Here's how the part is built. I have some questions about the finished solid (model axes, mm). A direction names the side the tool comes from. Round coordinates to 2 decimals unless told otherwise and drop trailing zeros. Loops run counter-clockwise (first coordinate to the right, second up) from the corner with the lowest first, then second, coordinate; pieces in that order, holes last. Notation, with made-up numbers: M -11.75,46.25 L 34.25,46.25 A23 ccw 34.25,82.25 Z; hole C 57,84 d6. An arc over 180 degrees is marked long. Use a Markdown table: item, result.
Autodesk Inventor part; units mm, degrees
ref_plane "YZ Plane" through (0, 0, 0) normal (1, 0, 0) x (0, 1, 0)
ref_plane "XZ Plane" through (0, 0, 0) normal (0, 1, 0) x (-1, 0, 0)
ref_plane "XY Plane" through (0, 0, 0) normal (0, 0, 1) x (1, 0, 0)
sketch "Sketch1" plane through (0, 0, 0) normal (0, 1, 0) x (-1, 0, 0)
  line L0 (6.6, -20) -> (-6.6, -20)
  line L1 (-6.6, -20) -> (-6.6, 20)
  line L2 (-6.6, 20) -> (6.6, 20)
  line L3 (6.6, 20) -> (6.6, -20)
  point P0 (0, 0)
  point P1 (0, -20)
  point P2 (-6.6, 0)
  dimension "d0" = 13.2
  dimension "d1" = 40
extrude "Extrusion1" add sketch "Sketch1" along normal blind 4.5
sketch "Sketch2" plane through (0, 0, 0) normal (0, -1, 0) x (1, 0, 0)
  line L0 (6.6, 20) -> (6.6, -20)
  circle A0 centre (6.6, 0) radius 2.05
  line L1 (-6.6, -20) -> (-6.6, 20)
  circle A1 centre (-6.6, 0) radius 2.05
  circle A2 centre (6.6, 0) radius 3.5
  circle A3 centre (-6.6, 0) radius 3.5
  point P0 (0, 0)
  dimension "d4" = 4.1
  dimension "d5" = 7
extrude "Extrusion2" add sketch "Sketch2" against normal blind 4.5
extrude "Extrusion3" cut sketch "Sketch2" against normal blind 3.1 contours A0 L0 | L0 A0 | A1 L1 | L1 A1
fillet "Fillet1" radius 2 8 edges at (6.6, 2.25, -20) (-6.6, 2.25, -20) (6.6, 2.25, 20) (-6.6, 2.25, 20) (6.6, 2.25, -3.5) (6.6, 2.25, 3.5) (-6.6, 2.25, -3.5) (-6.6, 2.25, 3.5)
fillet "Fillet2" radius 0.5 24 edges at (-6.6, 0, -11.5617) (-6.0142, 0, -19.4142) (0, 0, -20) (6.0142, 0, -19.4142) (6.6, 0, -11.5617) (10.1, 0, 0) (6.0142, 0, 19.4142) (6.6, 0, 11.5617) (0, 0, 20) (-6.0142, 0, 19.4142) (-6.6, 0, 11.5617) (-10.1, 0, 0) (-6.0142, 4.5, -19.4142) (-6.0142, 4.5, 19.4142) (-6.6, 4.5, 11.5617) (0, 4.5, 20) (6.0142, 4.5, 19.4142) (6.6, 4.5, 11.5617) (6.0142, 4.5, -19.4142) (10.1, 4.5, 0) (6.6, 4.5, -11.5617) (0, 4.5, -20) (-6.6, 4.5, -11.5617) (-10.1, 4.5, 0)
chamfer "Chamfer1" distance 0.25 angle 45 2 edges at (-8.65, 0, 0) (4.55, 0, 0)
properties part number "FuselageLock"
1. Imagine slicing it at A-A, the plane y = 2.55. Write out the boundary of the cut face in (x, z), then the cut area to 3 significant figures.
Answer sheet:
| item | result |
|---|---|
| outline | M -7.87,-3.26 A2 cw -6.6,-5.12 L -6.6,-18 A2 ccw -4.6,-20 L 4.6,-20 A2 ccw 6.6,-18 L 6.6,-5.12 A2 cw 7.87,-3.26 A3.5 ccw 7.87,3.26 A2 cw 6.6,5.12 L 6.6,18 A2 ccw 4.6,20 L -4.6,20 A2 ccw -6.6,18 L -6.6,5.12 A2 cw -7.87,3.26 A3.5 ccw Z; hole C -6.6,0 d4.1; hole C 6.6,0 d4.1 |
| area | 538 mm2 |
2. For pin 1 Ø1.2 at (x, z) = (6, 1) entering from -Y; pin 2 Ø1 at (y, z) = (1.5, -12.5) entering from -X; pin 3 Ø4.5 at (x, z) = (6.6, 0) entering from -Y, each with a flat end and sliding along its axis, tell me the tip position at first contact or that it passes through.
Answer sheet:
| item | result |
|---|---|
| pin 1 | y = 3.1 |
| pin 2 | x = -6.6 |
| pin 3 | y = 0.05 |
3. Which directions (+Z, -Z, +X, -X, +Y, -Y) give clear straight access to the entire face, cutting with the end or side of a thin tool? Please do faces 4 (the face through (6.6, 2, 11)), 5 (the face through (0, 4.5, 0)), 6 (the face through (4.55, 1.66, 0.09)).
Answer sheet:
| item | result |
|---|---|
| face 4 | +Z, +X, +Y, -Y |
| face 5 | +Z, -Z, +X, -X, +Y |
| face 6 | -Y |
4. Imagine slicing it at C-C, the plane z = 5.5. Write out the boundary of the cut face in (x, y), then the cut area to 3 significant figures.
Answer sheet:
| item | result |
|---|---|
| outline | M -6.6,0.5 A0.5 ccw -6.1,0 L 6.1,0 A0.5 ccw 6.6,0.5 L 6.6,4 A0.5 ccw 6.1,4.5 L -6.1,4.5 A0.5 ccw -6.6,4 Z |
| area | 59.2 mm2 |
5. Imagine slicing it at B-B, the plane z = 0. Write out the boundary of the cut face in (x, y), then the cut area to 3 significant figures.
Answer sheet:
| item | result |
|---|---|
| outline | M -10.1,0.5 A0.5 ccw -9.6,0 L -8.9,0 L -8.65,0.25 L -8.65,3.1 L -4.55,3.1 L -4.55,0.25 L -4.3,0 L 4.3,0 L 4.55,0.25 L 4.55,3.1 L 8.65,3.1 L 8.65,0.25 L 8.9,0 L 9.6,0 A0.5 ccw 10.1,0.5 L 10.1,4 A0.5 ccw 9.6,4.5 L -9.6,4.5 A0.5 ccw -10.1,4 Z |
| area | 65.1 mm2 |
6. I need wall thicknesses on probe 1 along X at (y, z) = (1.35, 0); probe 2 along X at (y, z) = (4, -14); probe 3 along Z at (x, y) = (5.5, 0.35). Which ranges of each line are inside material? Lowest first, please. Write a range as from..to.
Answer sheet:
| item | result |
|---|---|
| probe 1 | -10.1..-8.65, -4.55..4.55, 8.65..10.1 |
| probe 2 | -6.6..6.6 |
| probe 3 | -19.76..-1.73, 1.73..19.76 |
7. We'd pull the mould along Z, two halves only. Please class faces 1 (the face through (-6.03, 2.27, 19.4)), 2 (the face through (-8.65, 1.66, 0.09)), 3 (the face through (-10.1, 2.2, 0.1)): +Z half, -Z half, draft (parallel to the pull), parting line (faces both ways), or undercut.
Answer sheet:
| item | result |
|---|---|
| face 1 | +Z half |
| face 2 | undercut |
| face 3 | parting line |
